The listing builds one solid part. Answer for the finished solid, in the listing's coordinates (mm). Face numbers are marked on the shaded views. A direction names the side the tool comes from. Give positions to 0.01 mm unless a question says otherwise; leave off trailing zeros. Write each loop counter-clockwise with the first axis right and the second up, starting at its lowest first coordinate (ties: lowest second). Pieces come first, ordered by that corner, then holes. Notation, with made-up numbers: M -25,66.5 L -1,66.5 A16 cw -1,96.5 Z; hole C 67,-20.75 d5. An arc over 180 degrees is marked long. Return JSON: item names as keys, results as strings.
from build123d import *

# Parameters (mm, degrees)
F1_DEPTH = 76.2
F2_DEPTH = 25.4
F3_DEPTH = 74.93
F5_DEPTH = 76.94354


with BuildPart() as f1:
    # F0 (on Top) → F1 (new body)
    with BuildSketch(Plane.XY):
        with BuildLine():
            ThreePointArc((41.615028, -63.304463), (86.378043, -44.763015), (104.919491, 0))
            ThreePointArc((104.919491, 0), (86.378043, 44.763015), (41.615028, 63.304463))
            ThreePointArc((41.615028, 63.304463), (1.13027, 48.666615), (-20.631962, 11.522469))
            ThreePointArc((-20.631962, 11.522469), (-21.681366, -1.010742), (-20.232328, -13.504057))
            ThreePointArc((-20.232328, -13.504057), (1.912459, -49.306805), (41.615028, -63.304463))
        make_face()
        with BuildLine():
            ThreePointArc((-4.955136, -13.504057), (34.795208, 48.00656), (90.103581, 0))
            ThreePointArc((90.103581, 0), (48.434848, -48.00656), (-4.955136, -13.504057))
        make_face(mode=Mode.SUBTRACT)
    extrude(amount=F1_DEPTH)

    # F0 (on Top) → F2 (join)
    with BuildSketch(Plane.XY):
        with BuildLine():
            ThreePointArc((-20.631962, 11.522469), (1.13027, 48.666615), (41.615028, 63.304463))
            Line((41.615028, 63.304463), (41.615028, 63.438483))
            Line((41.615028, 63.438483), (-124.193631, 63.438483))
            Line((-124.193631, 63.438483), (-124.193631, -63.304463))
            Line((-124.193631, -63.304463), (41.615028, -63.304463))
            ThreePointArc((41.615028, -63.304463), (1.912459, -49.306805), (-20.232328, -13.504057))
            Line((-20.232328, -13.504057), (-84.665962, -13.504057))
            Line((-84.665962, -13.504057), (-84.665962, 11.522469))
            Line((-84.665962, 11.522469), (-20.631962, 11.522469))
        make_face()
    extrude(amount=F2_DEPTH)

    # F0 (on Top) → F3 (join)
    with BuildSketch(Plane.XY):
        with BuildLine():
            ThreePointArc((-20.232328, -13.504057), (-21.681366, -1.010742), (-20.631962, 11.522469))
            Line((-20.631962, 11.522469), (-84.665962, 11.522469))
            Line((-84.665962, 11.522469), (-84.665962, -13.504057))
            Line((-84.665962, -13.504057), (-20.232328, -13.504057))
        make_face()
    extrude(amount=F3_DEPTH)

    # F4 (on face) → F5 (cut, through all)
    with BuildSketch(Plane.XZ.offset(13.504057)):
        Polygon((-84.665962, 25.4), (-20.232328, 74.93), (-84.665962, 74.93), align=None)
    extrude(amount=-F5_DEPTH, mode=Mode.SUBTRACT)


solid = f1.part
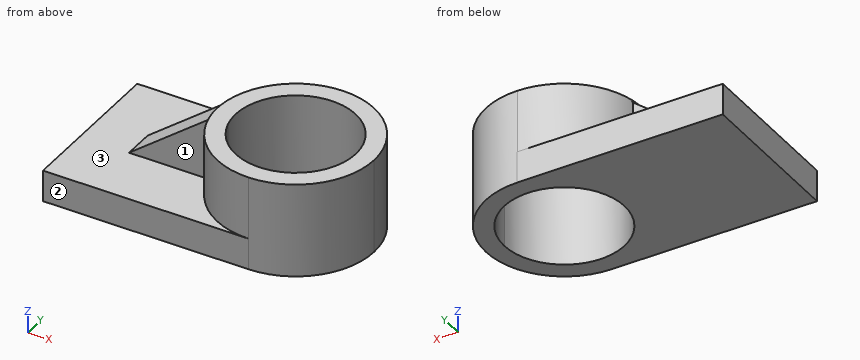
Item 1: Given pin 1 Ø4 at (x, z) = (-35.5, 44) entering from -Y; pin 2 Ø5 at (y, z) = (-28.5, 20.5) entering from +X; pin 3 Ø8 at (x, z) = (36.5, 36.5) entering from +Y, each flat-ended and moving along its own axis, determine where each tip first touches the part or whether it passes through.
Geometry results:
{"pin 1": "stops at y = -13.5", "pin 2": "stops at x = 99.33", "pin 3": "stops at y = 63.29"}
Item 2: Which of the six approach directions +Z, -Z, +X, -X, +Y, -Y give full straight-line access (tool end or side, diameter ignored) to the marked faces 1, 2 and 3?
Geometry results:
{"face 1": "+Z, -X, -Y", "face 2": "+Z, -Z, +X, -X, -Y", "face 3": "+Z, -X"}
Item 3: Find the intervals of material crossed by line 1 (X direction, y = -39.5, z = 7); line 2 (Y direction, x = -26, z = 43.5); line 3 (Y direction, x = 84, z = 69), in increasing order.
Geometry results:
{"line 1": "x = -124.19 to 13.49, 69.74 to 91.08", "line 2": "y = -13.5 to 11.52", "line 3": "y = -47.02 to -23.55, 23.55 to 47.02"}
Item 4: A cutting plane is placed at B-B, the plane x = 81.5. Write down the section's boundary in (y, z), plus the area to 3 significant figures.
Geometry results:
{"outline": "M -49.16,0 L -27.57,0 L -27.57,76.2 L -49.16,76.2 Z; M 27.57,0 L 49.16,0 L 49.16,76.2 L 27.57,76.2 Z", "area": "3,290 mm2"}
Item 5: A cutting plane is placed at C-C, the plane y = 40.5. Write down the section's boundary in (x, z), plus the area to 3 significant figures.
Geometry results:
{"outline": "M -124.19,0 L 14.95,0 L 14.95,76.2 L -7.04,76.2 L -7.04,25.4 L -124.19,25.4 Z; M 68.28,0 L 90.27,0 L 90.27,76.2 L 68.28,76.2 Z", "area": "6,330 mm2"}
Item 6: A cutting plane is placed at A-A, the plane z = 11.5. Write down the section's boundary in (x, y), plus the area to 3 significant figures.
Geometry results:
{"outline": "M -124.19,-63.3 L 41.62,-63.3 A63.3 ccw 41.62,63.3 L 41.62,63.44 L -124.19,63.44 Z; hole C 41.62,0 d96.98", "area": "19,900 mm2"}
Item 7: A cutting plane is placed at D-D, the plane x = -45.5. Write down the section's boundary in (y, z), plus the area to 3 significant figures.
Geometry results:
{"outline": "M -63.3,0 L 63.44,0 L 63.44,25.4 L 11.52,25.4 L 11.52,55.51 L -13.5,55.51 L -13.5,25.4 L -63.3,25.4 Z", "area": "3,970 mm2"}
